Part model, mm, in its own coordinate system. A direction names the side the tool comes from. Give positions to 0.01 mm unless a question says otherwise; leave off trailing zeros. Order: outer loops, then holes, each group sorted by start corner. A loop starts at its lowest first (then second) coordinate and runs counter-clockwise, first axis right, second up. Notation, with made-up numbers: (28, 22) -> (68, 22) arc R24 ccw to (68, 44) -> close; hole circle Ø4 at (-2.5, -37.5). An arc over 180 degrees is marked (long way). Write item = value, one per line. Start each with the question number.
(1) Probe line 1 along Y through (x, z) = (-9, 0.65); line 2 along Y through (x, z) = (8.5, 5). List the from-to ranges inside material, lowest first. Write a range as from..to.
(2) Saw through at B-B, the plane z = 4.2. List the corners of the cut face in (x, y).
(3) Flat gauge pins, fed straight in: pin 1 (2 mm diameter, centred on x = -1.5, y = 5.5, fed in from +Z); pin 2 (3 mm diameter, centred on x = 3, z = 2, fed in from +Y); pin 3 (1.2 mm diameter, centred on x = 9, z = 3.5, fed in from +Y); pin 4 (1.8 mm diameter, centred on x = -4, z = 4, fed in from +Y). Where does each tip first touch, or does it go through?
(4) Saw through at C-C, the plane x = -4.25. List the corners of the cut face in (y, z), then the cut area to 3 significant figures.
(5) Two-plate mould, pull along X, no slides. Class faces 1 (the cylindrical face through (4.88, -3.49, 2.96)), 2 (the flat face through (0, -1, 0)), 3 (the cylindrical face through (-5.54, -3.11, 2.96)), 4 (the flat face through (-9.75, -1, 3)): pulls with the +X half, pulls with the -X half, needs draft (parallel to the pull), parting line crosses it, or undercut.
(6) Saw through at D-D, the plane x = -6.75. List the corners of the cut face in (y, z) (3 decimals), then the cut area to 3 significant figures.
(7) Saw through at A-A, the plane y = -2.5. List the corners of the cut face in (x, z).
(8) Which spindle directions (+Z, -Z, +X, -X, +Y, -Y) get a long thin tool onto all of the face, cutting with end or side? Do faces 5 (the flat face through (0, -1, 6)), 6 (the flat face through (8, 5, 3)), 7 (the flat face through (-5, 4, 3)). Say none if no direction does.
from build123d import *

# Parameters (mm, degrees)
SKETCH1_R           = 1
BOSS_EXTRUDE1_DEPTH = 6
BOSS_EXTRUDE2_DEPTH = 6


with BuildPart() as part:
    # Sketch1 → Boss-Extrude1 (new body)
    with BuildSketch(Plane.XY):
        Polygon((-9.75, 4), (0.25, 4), (0.25, 5), (9.75, 5), (9.75, -5), (-9.75, -5), align=None)
        with Locations((-4.75, -2.5)):
            Circle(SKETCH1_R, mode=Mode.SUBTRACT)
        with Locations(Location((4.75, -2.5, 0), (0, 0, 180))):
            Circle(SKETCH1_R, mode=Mode.SUBTRACT)
    extrude(amount=BOSS_EXTRUDE1_DEPTH)

    # Sketch2 → Boss-Extrude2 (add)
    with BuildSketch(Plane(origin=(0, 0, 0), x_dir=(-1, 0, 0), z_dir=(0, 0, -1))):
        Polygon((-7.25, 5), (8.75, 10), (8.779827499, 9.904552002), (-6.914738908, 5), align=None)
    extrude(amount=-BOSS_EXTRUDE2_DEPTH)


solid = part.part
Results list:
q1.line_1 = -5..4
q1.line_2 = -5..5
q2.outline = (-9.75, -5) -> (9.75, -5) -> (9.75, 5) -> (7.25, 5) -> (-8.75, 10) -> (-8.78, 9.9) -> (6.91, 5) -> (0.25, 5) -> (0.25, 4) -> (-9.75, 4) -> close; hole circle Ø2 at (-4.75, -2.5); hole circle Ø2 at (4.75, -2.5)
q3.pin_1 = through
q3.pin_2 = 6.8
q3.pin_3 = 5
q3.pin_4 = 8.8
q4.outline = (-5, 0) -> (-3.37, 0) -> (-3.37, 6) -> (-5, 6) -> close; (-1.63, 0) -> (4, 0) -> (4, 6) -> (-1.63, 6) -> close; (8.49, 0) -> (8.59, 0) -> (8.59, 6) -> (8.49, 6) -> close
q4.area = 44.2 mm^2
q5.face_1 = undercut
q5.face_2 = needs draft
q5.face_3 = undercut
q5.face_4 = pulls with the -X half
q6.outline = (-5, 0) -> (4, 0) -> (4, 6) -> (-5, 6) -> close; (9.27, 0) -> (9.375, 0) -> (9.375, 6) -> (9.27, 6) -> close
q6.area = 54.6 mm^2
q7.outline = (-9.75, 0) -> (-5.75, 0) -> (-5.75, 6) -> (-9.75, 6) -> close; (-3.75, 0) -> (3.75, 0) -> (3.75, 6) -> (-3.75, 6) -> close; (5.75, 0) -> (9.75, 0) -> (9.75, 6) -> (5.75, 6) -> close
q8.face_5 = +Z, +X, -X, +Y, -Y
q8.face_6 = +Z, -Z, +X, +Y
q8.face_7 = +Z, -Z, -X
